Answer from the drawing. Dimensions are ordinates in mm from the lowest x, y and z of the part. Give positions to 0.01 mm unless a question says otherwise; leave off trailing zeros. Loops run counter-clockwise (first coordinate to the right, second up) from the corner with the lowest first, then second, coordinate; pieces in that order, holes last.
Item 1: Section C-C, the plane z = 171.5 is taken. Give the vertices of the cut face in (x, y) (1 decimal).
Item 2: Section B-B, the plane x = 10 is taken. Give the vertices of the cut face in (y, z) (1 decimal).
Item 3: Consider line 1 along X through (y, z) = (0.4, 75) (1 decimal); line 2 along X through (y, z) = (1.6, 150) (1 decimal). Determine where each line is inside the solid, lowest interval first.
Item 4: This flat-tipped pin is pushed along its axis until it touches: pin 1 Ø4 at (x, z) = (21.31, 200.44) entering from -Y. Where does it stop, or does it pass through?
Item 5: Section A-A, the plane y = 0.6 is taken. Give the number of separate pieces and of enclosed holes in the cut face, and give its area (3 significant figures).
Item 6: Section D-D, the plane z = 125.5 is taken. Give the vertices of the cut face in (x, y) (1 decimal).
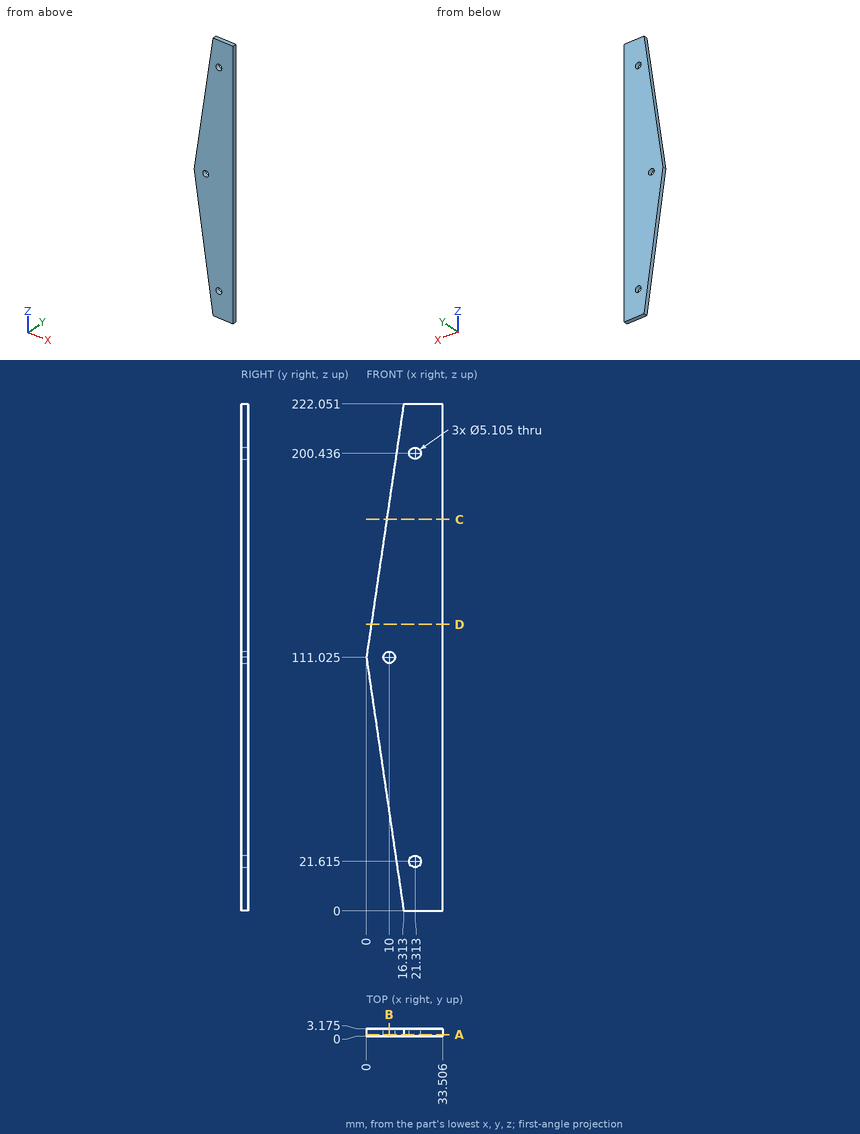
Worked answers:
1. outline: (8.9, 0) - (33.5, 0) - (33.5, 3.2) - (8.9, 3.2) - close
2. outline: (0, 43) - (3.2, 43) - (3.2, 108.5) - (0, 108.5) - close; (0, 113.6) - (3.2, 113.6) - (3.2, 179.1) - (0, 179.1) - close
3. line 1: x = 5.3 to 33.5
3. line 2: x = 5.7 to 33.5
4. pin 1: passes through
5. separate pieces: 1
5. enclosed holes: 3
5. area: 5,570 mm2
6. outline: (2.1, 0) - (33.5, 0) - (33.5, 3.2) - (2.1, 3.2) - close
